```python
from build123d import *

# Parameters (mm, degrees)
EXTRUDE_1_DEPTH = 1.6
SKETCH_2_W      = 3.67331973
SKETCH_2_H      = 3.463876061
SKETCH_2_W_2    = 3.496098164
SKETCH_2_H_2    = 3.077210826
SKETCH_2_W_3    = 3.318876597
SKETCH_2_H_3    = 3.173877135
SKETCH_2_W_4    = 2.321089706
SKETCH_2_H_4    = 1.877636292
EXTRUDE_2_DEPTH = 0.95


with BuildPart() as part:
    # 스케치1 → 보스-돌출1 (new body)
    with BuildSketch(Plane(origin=(0, 0, 0), x_dir=(1, 0, 0), z_dir=(0, 1, 0))):
        Polygon((0, 10.6), (1.5, 12.1), (12.1, 12.1), (12.1, 0), (0, 0), align=None)
    extrude(amount=EXTRUDE_1_DEPTH)

    # 스케치2 → 보스-돌출2 (add)
    with BuildSketch(Plane(origin=(0, 1.6, 0), x_dir=(1, 0, 0), z_dir=(0, 1, 0))):
        with Locations((3.955563312, 8.386102459)):
            Rectangle(SKETCH_2_W, SKETCH_2_H)
        with Locations((8.78082322, 8.563324025)):
            Rectangle(SKETCH_2_W_2, SKETCH_2_H_2)
        with Locations((4.728893782, 3.343343358)):
            Rectangle(SKETCH_2_W_3, SKETCH_2_H_3)
        with Locations((9.60999322, 2.63077873)):
            Rectangle(SKETCH_2_W_4, SKETCH_2_H_4)
    extrude(amount=EXTRUDE_2_DEPTH)


solid = part.part
```
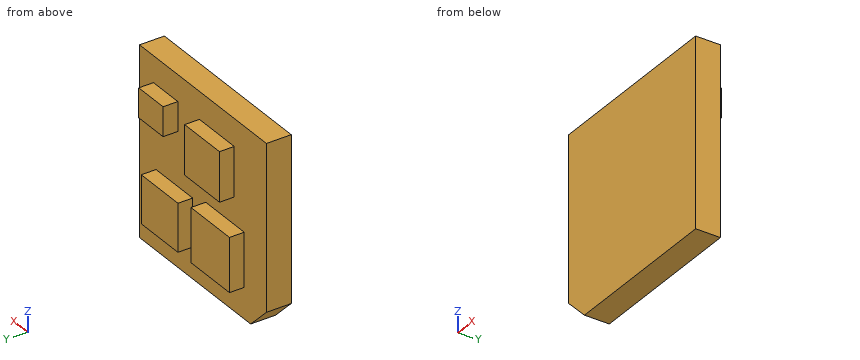
Geometry check sheet. Reference: the model listing, model coordinates, mm. Give positions to 0.01 mm unless a question says otherwise; leave off trailing zeros. Write each loop counter-clockwise with the first axis right and the second up, starting at its lowest first coordinate (ties: lowest second). Pieces come first, ordered by that corner, then holes.
1) Material ranges on L1, parallel to X at y = 2.4, z = -9.5; L2, parallel to Z at x = 9.25, y = 1.75; L3, parallel to Y at x = 8.5, z = -10.5, recorded low to high.
2) Gauge pin test, flat ends, axial feed: pin 1 (1 mm diameter, centred on y = 2.5, z = -8.5, fed in from -X); pin 2 (0.5 mm diameter, centred on x = 9.5, y = 2, fed in from -Z); pin 3 (0.5 mm diameter, centred on y = 2, z = -8.5, fed in from +X); pin 4 (1 mm diameter, centred on x = 10, y = 2, fed in from +Z). Record the tip position at first contact, or that the pin passes through.
3) Section check B-B, the plane z = -7.5. Record the boundary of the cut face in (x, y), and give its area (3 significant figures).
4) Section check A-A, the plane y = 2.15. Record the boundary of the cut face in (x, z).
5) Section check C-C, the plane x = 7.25. Record the boundary of the cut face in (y, z), and give its area (3 significant figures).
6) Section check D-D, the plane z = -3.25. Record the boundary of the cut face in (x, y).
Computed:
1. L1: x = 2.12 to 5.79, 7.03 to 10.53
1. L2: z = -10.1 to -7.02, -3.57 to -1.69
1. L3: y = 0 to 1.6
2. pin 1: stops at x = 2.12
2. pin 2: stops at z = -10.1
2. pin 3: stops at x = 10.53
2. pin 4: stops at z = 0
3. outline: (0, 0) - (12.1, 0) - (12.1, 1.6) - (10.53, 1.6) - (10.53, 2.55) - (7.03, 2.55) - (7.03, 1.6) - (5.79, 1.6) - (5.79, 2.55) - (2.12, 2.55) - (2.12, 1.6) - (0, 1.6) - close
3. area: 26.2 mm2
4. outline: (2.12, -10.12) - (5.79, -10.12) - (5.79, -6.65) - (2.12, -6.65) - close; (3.07, -4.93) - (6.39, -4.93) - (6.39, -1.76) - (3.07, -1.76) - close; (7.03, -10.1) - (10.53, -10.1) - (10.53, -7.02) - (7.03, -7.02) - close; (8.45, -3.57) - (10.77, -3.57) - (10.77, -1.69) - (8.45, -1.69) - close
5. outline: (0, -12.1) - (1.6, -12.1) - (1.6, -10.1) - (2.55, -10.1) - (2.55, -7.02) - (1.6, -7.02) - (1.6, 0) - (0, 0) - close
5. area: 22.3 mm2
6. outline: (0, 0) - (12.1, 0) - (12.1, 1.6) - (10.77, 1.6) - (10.77, 2.55) - (8.45, 2.55) - (8.45, 1.6) - (6.39, 1.6) - (6.39, 2.55) - (3.07, 2.55) - (3.07, 1.6) - (0, 1.6) - close
